Work out the finished part from the listing and answer in its coordinate system (mm). Face numbers are marked on the shaded views. A direction names the side the tool comes from. Round coordinates to 2 decimals unless told otherwise and drop trailing zeros. Order: outer loops, then holes, each group sorted by start corner. A loop starts at its lowest first (then second) coordinate and runs counter-clockwise, first axis right, second up. Notation, with made-up numbers: (38, 52.25) - (93, 52.25) arc R31 cw to (93, 87.25) - close; hole circle Ø10 at (83, 78.5). An arc over 180 degrees is marked (long way). Answer in a Markdown table with one row per item.
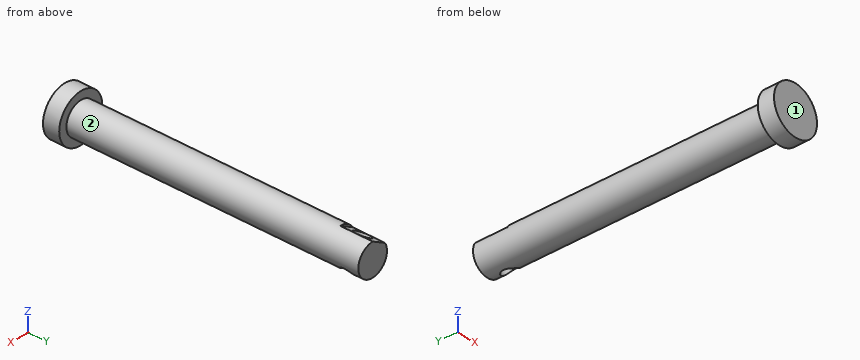
from build123d import *

# Parameters (mm, degrees)
SKETCH_1_R          = 7.5
EXTRUDE_1_DEPTH     = 5
SKETCH_2_R          = 5
EXTRUDE_2_DEPTH     = 90
CUT_EXTRUDE_1_DEPTH = 10
SKETCH_13_R         = 2.500883101
CUT_EXTRUDE_2_DEPTH = 10


with BuildPart() as part:
    # Эскиз1 → Бобышка-Вытянуть1 (new body)
    with BuildSketch(Plane(origin=(0, 0, 0), x_dir=(1, 0, 0), z_dir=(0, 1, 0))):
        with Locations((40.81014851, -30.211534636)):
            Circle(SKETCH_1_R)
    extrude(amount=EXTRUDE_1_DEPTH)

    # Эскиз2 → Бобышка-Вытянуть2 (add)
    with BuildSketch(Plane(origin=(0, 5, 0), x_dir=(1, 0, 0), z_dir=(0, 1, 0))):
        with Locations((40.81014851, -30.211534636)):
            Circle(SKETCH_2_R)
    extrude(amount=EXTRUDE_2_DEPTH)

    # Эскиз12 → Вырез-Вытянуть1 (cut)
    with BuildSketch(Plane(origin=(0, 95, 0), x_dir=(1, 0, 0), z_dir=(0, 1, 0))):
        Polygon((40.81014851, -35.211534636), (36.479002075, -32.709768123), (36.139784444, -33.297033651), (40.47093088, -35.798800164), align=None)
    extrude(amount=-CUT_EXTRUDE_1_DEPTH, mode=Mode.SUBTRACT)

    # Эскиз13 → Вырез-Вытянуть2 (cut)
    with BuildSketch(Plane(origin=(-5.040884978, 0, 8.726957886), x_dir=(0.865923408, 0, 0.50017662), z_dir=(-0.50017662, 0, 0.865923408))):
        with Locations((50.449566166, 90)):
            Circle(SKETCH_13_R)
    extrude(amount=-CUT_EXTRUDE_2_DEPTH, mode=Mode.SUBTRACT)


solid = part.part
1) Find section B-B, the plane z = 36.75. Give the vertices of the cut face in (x, y), then the cut area to 3 significant figures.
Filled in:
| item | result |
|---|---|
| outline | (37.14, 0) - (44.48, 0) - (44.48, 5) - (37.14, 5) - close |
| area | 36.7 mm^2 |
2) Find the intervals of material crossed by probe 1 along Y at (x, z) = (45.5, 32.25); probe 2 along Y at (x, z) = (42.25, 29.75); probe 3 along Y at (x, z) = (40.5, 33.75), in increasing order. Write a range as from..to.
Filled in:
| item | result |
|---|---|
| probe 1 | y = 0..5 |
| probe 2 | y = 0..87.71, 92.29..95 |
| probe 3 | y = 0..88, 92..95 |
3) Find section D-D, the plane z = 24.25. Give the vertices of the cut face in (x, y).
Filled in:
| item | result |
|---|---|
| outline | (36.26, 0) - (45.36, 0) - (45.36, 5) - (36.26, 5) - close |
4) Each of these flat-tipped pins is pushed along its axis until it touches: pin 1 (1 mm diameter, centred on y = 72.5, z = 29, fed in from -X); pin 2 (1.5 mm diameter, centred on y = 60, z = 34.5, fed in from +X); pin 3 (3 mm diameter, centred on y = 29, z = 34.5, fed in from -X). Where does it stop, or does it pass through?
Filled in:
| item | result |
|---|---|
| pin 1 | stops at x = 35.86 |
| pin 2 | stops at x = 44.34 |
| pin 3 | stops at x = 36.66 |
5) Which of the six approach directions +Z, -Z, +X, -X, +Y, -Y give full straight-line access (tool end or side, diameter ignored) to the marked faces 1 and 2?
Filled in:
| item | result |
|---|---|
| face 1 | +Z, -Z, +X, -X, -Y |
| face 2 | +Y |
6) Find section C-C, the plane y = 64. Give the vertices of the cut face in (x, z), then the cut area to 3 significant figures.
Filled in:
| item | result |
|---|---|
| outline | circle Ø10 at (40.81, 30.21) |
| area | 78.5 mm^2 |
7) Find section A-A, the plane y = 86. Give the vertices of the cut face in (x, z).
Filled in:
| item | result |
|---|---|
| outline | (36.48, 32.71) arc R5 ccw (long way) to (40.81, 35.21) - close |
